Part model, mm, in its own coordinate system. A direction names the side the tool comes from. Round coordinates to 2 decimals unless told otherwise and drop trailing zeros. Loops run counter-clockwise (first coordinate to the right, second up) from the corner with the lowest first, then second, coordinate; pieces in that order, holes last. Notation, with made-up numbers: (77.25, 19) - (83.25, 19) arc R18 ccw to (83.25, 44) - close; hole circle Ø3 at (23.25, 49.5). An arc over 180 degrees is marked (long way). Write each question's results on one line, items separated by ' | '. Start each with the question number.
(1) Cut at A-A, the plane z = 45. List the corners of the cut face in (x, y).
(2) Drill centre lines: L1, parallel to X at y = 75, z = 19.5; L2, parallel to X at y = 75, z = 4.5 (3 decimals); L3, parallel to Y at x = 0, z = 20. Where is each one in solid material? Low to high.
(3) Tool access for faces 1 (the face through (81.846, -1.421, 42.395)), 2 (the face through (-1, 2, 0)), 3 (the face through (-1.87, 83.42, 4.93)): list every direction of +Z, -Z, +X, -X, +Y, -Y with a clear straight run to the whole face (end or side of a thin tool).
(4) Mould opens along X. For faces 4 (the face through (-1.18, -144.99, 42.4)), 5 (the face through (-83.846, 1.432, 42.395)), 6 (the face through (83.846, -1.432, 42.395)), 7 (the face through (6, 75, 10)) say: released by +X, released by -X, zero draft, split by the parting line, or undercut.
(5) Cut at B-B, the plane z = 5. Give the number of separate pieces and of enclosed holes in the cut face, then the cut area to 3 significant figures.
(6) Flat gauge pins, fed straight in: P1, Ø5, axis at y = 87.5, z = 23, coming from the -X side; P2, Ø14, axis at x = 0, y = 75, coming from the -Z side; P3, Ø2, axis at y = -91.5, z = 27, coming from the -X side; P4, Ø6.5, axis at x = 0, y = 75, coming from the +Z side. Where does each tip first touch, or does it go through?
from build123d import *

# Parameters (mm, degrees)
F1_DEPTH       = 50
F2_R           = 35
F3_T           = -2
F4_R           = 10
F5_DEPTH       = 30
F5_TAPER       = 3
F7_D           = 11
F7_CBORE_D     = 17.25
F7_CBORE_DEPTH = 10


with BuildPart() as f1:
    # F0 (on Top) → F1 (new body)
    with BuildSketch(Plane.XY):
        with BuildLine():
            ThreePointArc((65.3834841531, 100), (0, 145), (-65.3834841531, 100))
            ThreePointArc((-65.3834841531, 100), (-83.8495475407, 0), (-65.3834841531, -100))
            ThreePointArc((-65.3834841531, -100), (0, -145), (65.3834841531, -100))
            ThreePointArc((65.3834841531, -100), (83.8495475407, 0), (65.3834841531, 100))
        make_face()
    extrude(amount=F1_DEPTH)

    # F2
    f2_edges = [f1.edges().sort_by_distance(p)[0] for p in [
        (0, -145, 0),
    ]]
    fillet(f2_edges, radius=F2_R)

    # F3
    f3_openings = [f1.faces().sort_by_distance(p)[0] for p in [
        (0, 0, 50),
    ]]
    offset(amount=F3_T, openings=f3_openings)

    # F4 (on face) → F5 (join)
    with BuildSketch(Plane.XY.offset(2)):
        with Locations((0, 75)):
            Circle(F4_R)
    extrude(amount=F5_DEPTH, taper=F5_TAPER)

    # F7 (through all)
    with Locations(Plane(origin=(0, 0, 0), x_dir=(1, 0, 0), z_dir=(0, 0, -1))):
        with Locations((0, -75)):
            CounterBoreHole(F7_D / 2, F7_CBORE_D / 2, F7_CBORE_DEPTH)


solid = f1.part
A:
1) outline: (-65.38, -100) arc R70 ccw to (65.38, -100) arc R280 ccw to (65.38, 100) arc R70 ccw to (-65.38, 100) arc R280 ccw to start; hole (-63.52, -99.29) arc R68 ccw to (63.52, -99.29) arc R278 ccw to (63.52, 99.29) arc R68 ccw to (-63.52, 99.29) arc R278 ccw to start
2) L1: -69.86 to -67.52, -9.08 to -5.5, 5.5 to 9.08, 67.52 to 69.86 | L2: -55.061 to -50.289, -9.869 to -8.625, 8.625 to 9.869, 50.289 to 55.061 | L3: -141.62 to -139.39, 65.94 to 69.5, 80.5 to 84.06, 139.39 to 141.62
3) face 1: +Z | face 2: -Z, +X, -X, +Y, -Y | face 3: -Z
4) face 4: split by the parting line | face 5: released by -X | face 6: released by +X | face 7: undercut
5) separate pieces: 2 | enclosed holes: 2 | area: 2,750 mm2
6) P1: x = -68.79 | P2: z = 10 | P3: x = -67.92 | P4: through
